```python
from build123d import *

# Parameters (mm, degrees)
EXTRUDE_1_DEPTH     = 5
SKETCH_2_R          = 2
CUT_EXTRUDE_1_DEPTH = 15
FILLET_1_R          = 2


with BuildPart() as part:
    # 草图1 → 凸台-拉伸1 (new, symmetric)
    with BuildSketch(Plane.XY):
        with BuildLine():
            Line((0, 0), (20, 0))
            Line((20, 0), (20, 10))
            ThreePointArc((20, 10), (10, 4.633249581), (0, 10))
            Line((0, 10), (0, 0))
        make_face()
    extrude(amount=EXTRUDE_1_DEPTH, both=True)

    # 草图2 → 切除-拉伸1 (cut)
    with BuildSketch(Plane(origin=(0, 0, 0), x_dir=(1, 0, 0), z_dir=(0, 1, 0))):
        with Locations(Location((10, 0, 0), (0, 0, 90))):
            Circle(SKETCH_2_R)
    extrude(amount=CUT_EXTRUDE_1_DEPTH, mode=Mode.SUBTRACT)

    # 圆角1
    fillet_1_edges = [part.edges().sort_by_distance(p)[0] for p in [
        (20, 5, 5),
        (0, 5, 5),
        (20, 5, -5),
        (0, 5, -5),
    ]]
    fillet(fillet_1_edges, radius=FILLET_1_R)


solid = part.part
```
Here's how the part is built. I have some questions about the finished solid (model axes, mm). Give positions to 0.01 mm unless a question says otherwise; leave off trailing zeros. Order: outer loops, then holes, each group sorted by start corner. A loop starts at its lowest first (then second) coordinate and runs counter-clockwise, first axis right, second up. Notation, with made-up numbers: (-4.75, -4.5) - (18.25, -4.5) arc R35 cw to (18.25, 33.5) - close; hole circle Ø7 at (14.25, -10.75). An arc over 180 degrees is marked (long way). Answer as a JSON object with one key per item and string values. Group by question number.
Item 1: Please list where these lines run through material, in increasing order: probe 1 along Z at (x, y) = (10, 3.2); probe 2 along X at (y, z) = (1.4, 0); probe 3 along Y at (x, z) = (10, -3.75).
Item 2: If we mould it in two halves opening along X, with no side actions, what happens to faces 1 (the cylindrical face through (8, 2, 0)), 2 (the flat face through (10, 3, 5)), 3 (the cylindrical face through (0.6, 4.93, -4.43))? For each: pulls with the +X half, pulls with the -X half, needs draft (parallel to the pull), parting line crosses it, or undercut.
Item 3: If we section it at B-B on z = 0: Please give me the cut outline in (x, y).
Item 4: If we section it at A-A on x = 10: Please give me the cut outline in (y, z), and give its area (3 significant figures).
Item 5: If we section it at D-D on x = 14.75: Please give me the cut outline in (y, z), and give its area (3 significant figures).
Item 6: If we section it at C-C on x = 7: Please give me the cut outline in (y, z), and give its area (3 significant figures).
Item 7: For P1, Ø2, axis at x = 7, z = -2, coming from the -Y side; P2, Ø6, axis at x = 4, z = 3.5, coming from the +Y side; P3, Ø2, axis at x = 12, z = -1.5, coming from the +Y side, each with a flat end and sliding along its axis, tell me the tip position at first contact or that it passes through.
Result set:
{
 "1": {"probe 1": "-5 to -2, 2 to 5", "probe 2": "0 to 8, 12 to 20", "probe 3": "0 to 4.63"},
 "2": {"face 1": "undercut", "face 2": "needs draft", "face 3": "pulls with the -X half"},
 "3": {"outline": "(0, 0) - (8, 0) - (8, 4.8) arc R12 cw to (0, 10) - close; (12, 0) - (20, 0) - (20, 10) arc R12 cw to (12, 4.8) - close"},
 "4": {"outline": "(0, -5) - (4.63, -5) - (4.63, -2) - (0, -2) - close; (0, 2) - (4.63, 2) - (4.63, 5) - (0, 5) - close", "area": "27.8 mm²"},
 "5": {"outline": "(0, -5) - (5.61, -5) - (5.61, 5) - (0, 5) - close", "area": "56.1 mm²"},
 "6": {"outline": "(0, -5) - (5.01, -5) - (5.01, 5) - (0, 5) - close", "area": "50.1 mm²"},
 "7": {"P1": "y = 0", "P2": "y = 8.7", "P3": "y = 5.01"}
}
